from build123d import *

# Parameters (mm, degrees)
F0_R     = 12.7
F1_DEPTH = 6.35
F2_T     = -2.54


with BuildPart() as f1:
    # F0 (on Top) → F1 (new body)
    with BuildSketch(Plane.XY):
        with BuildLine():
            Line((-46.9330802516, 19.4403183641), (-58.6663503145, 24.3003979552))
            ThreePointArc((-58.6663503145, 24.3003979552), (-62.2798653056, 12.388235448), (-63.5, 0))
            Line((-63.5, 0), (-50.8, 0))
            ThreePointArc((-50.8, 0), (-50.0884898607, -8.4724957052), (-47.9738904144, -16.7076580798))
            Line((-47.9738904144, -16.7076580798), (-59.7227298995, -21.5741867367))
            ThreePointArc((-59.7227298995, -21.5741867367), (-53.5964944807, -34.0538658507), (-44.9012806053, -44.9012806053))
            Line((-44.9012806053, -44.9012806053), (-35.9210244843, -35.9210244843))
            ThreePointArc((-35.9210244843, -35.9210244843), (-28.2229678374, -42.238656305), (-19.4403183641, -46.9330802516))
            Line((-19.4403183641, -46.9330802516), (-24.3003979552, -58.6663503145))
            ThreePointArc((-24.3003979552, -58.6663503145), (-12.388235448, -62.2798653056), (0, -63.5))
            Line((0, -63.5), (0, -50.8))
            ThreePointArc((0, -50.8), (9.9105883584, -49.8238922445), (19.4403183641, -46.9330802516))
            Line((19.4403183641, -46.9330802516), (24.3003979552, -58.6663503145))
            ThreePointArc((24.3003979552, -58.6663503145), (35.2787097967, -52.7983203812), (44.9012806053, -44.9012806053))
            Line((44.9012806053, -44.9012806053), (35.9210244843, -35.9210244843))
            ThreePointArc((35.9210244843, -35.9210244843), (42.238656305, -28.2229678374), (46.9330802516, -19.4403183641))
            Line((46.9330802516, -19.4403183641), (58.6663503145, -24.3003979552))
            ThreePointArc((58.6663503145, -24.3003979552), (62.2798653056, -12.388235448), (63.5, 0))
            Line((63.5, 0), (50.8, 0))
            ThreePointArc((50.8, 0), (49.8238922445, 9.9105883584), (46.9330802516, 19.4403183641))
            Line((46.9330802516, 19.4403183641), (58.6663503145, 24.3003979552))
            ThreePointArc((58.6663503145, 24.3003979552), (52.7983203812, 35.2787097967), (44.9012806053, 44.9012806053))
            Line((44.9012806053, 44.9012806053), (35.9210244843, 35.9210244843))
            ThreePointArc((35.9210244843, 35.9210244843), (28.2229678374, 42.238656305), (19.4403183641, 46.9330802516))
            Line((19.4403183641, 46.9330802516), (24.3003979552, 58.6663503145))
            ThreePointArc((24.3003979552, 58.6663503145), (12.388235448, 62.2798653056), (0, 63.5))
            Line((0, 63.5), (0, 50.8))
            ThreePointArc((0, 50.8), (-9.9105883584, 49.8238922445), (-19.4403183641, 46.9330802516))
            Line((-19.4403183641, 46.9330802516), (-24.3003979552, 58.6663503145))
            ThreePointArc((-24.3003979552, 58.6663503145), (-35.2787097967, 52.7983203812), (-44.9012806053, 44.9012806053))
            Line((-44.9012806053, 44.9012806053), (-35.9210244843, 35.9210244843))
            ThreePointArc((-35.9210244843, 35.9210244843), (-42.238656305, 28.2229678374), (-46.9330802516, 19.4403183641))
        make_face()
        Circle(F0_R, mode=Mode.SUBTRACT)
    extrude(amount=F1_DEPTH)

    # F2
    f2_openings = [f1.faces().sort_by_distance(p)[0] for p in [
        (-34.280877, 51.304958, 6.35),
    ]]
    offset(amount=F2_T, openings=f2_openings, kind=Kind.INTERSECTION)


solid = f1.part
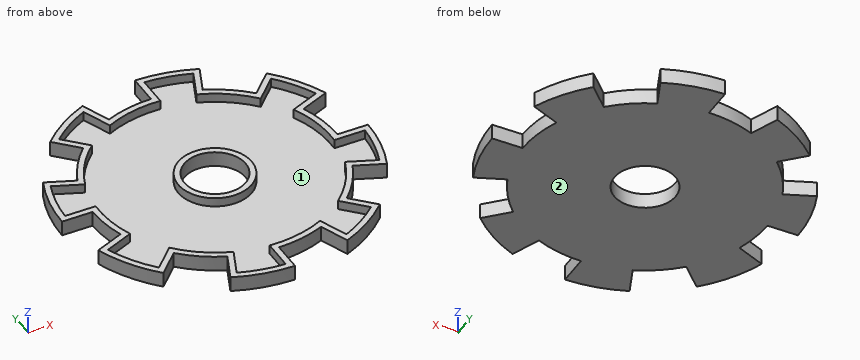
The listing builds one solid part. Answer for the finished solid, in the listing's coordinates (mm). Face numbers are marked on the shaded views. Coordinates: 2 decimals unless noted, no trailing zeros. Write each loop counter-clockwise with the first axis right and the second up, starting at its lowest first coordinate (ties: lowest second). Pieces come first, ordered by that corner, then holes. Notation, with made-up numbers: (0, 21.5) - (25, 21.5) arc R23 ccw to (25, 33.5) - close; hole circle Ø3 at (9.5, 59.25). An arc over 180 degrees is marked (long way). Answer as CSV lines item,"result".
1. Find section A-A (x = 7.5). Give the vertices of the cut face in (y, z).
Computed values:
outline,"(-50.24, 0) - (-10.25, 0) - (-10.25, 6.35) - (-13.27, 6.35) - (-13.27, 2.54) - (-47.67, 2.54) - (-47.67, 6.35) - (-50.24, 6.35) - close; (10.25, 0) - (63.06, 0) - (63.06, 6.35) - (60.5, 6.35) - (60.5, 2.54) - (13.27, 2.54) - (13.27, 6.35) - (10.25, 6.35) - close"
2. Determine the mould class of the marked faces 1 and 2 for opening direction X: +X half, -X half, draft (parallel to the pull), parting line (faces both ways), or undercut.
Computed values:
face 1,"undercut"
face 2,"draft"
3. Straight lines are drawn through the part: line 1 (X direction, y = -17, z = 4.5); line 2 (X direction, y = 6.5, z = 5.75); line 3 (X direction, y = 2, z = 5.25). For each, find the intervals that lie inside material, in ascending order. Write a range as [from, to].
Computed values:
line 1,"x = [-48.68, -45.17], [45.17, 47.68], [58.54, 61.18]"
line 2,"x = [-63.17, -60.61], [-13.78, -10.91], [10.91, 13.78], [47.82, 50.38]"
line 3,"x = [-63.47, -48.22], [-15.11, -12.54], [12.54, 15.11], [48.22, 50.76]"
4. Given P1, Ø3, axis at y = -53.5, z = 4, coming from the -X side; P2, Ø1, axis at y = -33.5, z = 5.5, coming from the -X side; P3, Ø1.9, axis at y = -56.5, z = 3.5, coming from the +X side, each flat-ended and moving along its own axis, determine where each tip first touches the part or whether it passes through.
Computed values:
P1,"stops at x = -22.78"
P2,"stops at x = -54.25"
P3,"stops at x = 30.76"
5. Find section B-B (y = 38). Give the vertices of the cut face in (x, z).
Computed values:
outline,"(-38, 0) - (33.71, 0) - (33.71, 6.35) - (29.75, 6.35) - (29.75, 2.54) - (-34.41, 2.54) - (-34.41, 6.35) - (-38, 6.35) - close; (38, 0) - (50.87, 0) - (50.87, 6.35) - (47.67, 6.35) - (47.67, 2.54) - (41.59, 2.54) - (41.59, 6.35) - (38, 6.35) - close"
